```python
from build123d import *

# Parameters (mm, degrees)
SKETCH1_R           = 3.15
BOSS_EXTRUDE1_DEPTH = 12
SKETCH2_R           = 2.1
BOSS_EXTRUDE2_DEPTH = 5


with BuildPart() as part:
    # Sketch1 → Boss-Extrude1 (new body)
    with BuildSketch(Plane(origin=(0, 0, 0), x_dir=(0, 0, -1), z_dir=(1, 0, 0))):
        with BuildLine():
            Line((-15.5, -6), (15.5, -6))
            ThreePointArc((15.5, -6), (16.914213562, -5.414213562), (17.5, -4))
            Line((17.5, -4), (17.5, 4))
            ThreePointArc((17.5, 4), (16.914213562, 5.414213562), (15.5, 6))
            Line((15.5, 6), (-15.5, 6))
            ThreePointArc((-15.5, 6), (-16.914213562, 5.414213562), (-17.5, 4))
            Line((-17.5, 4), (-17.5, -4))
            ThreePointArc((-17.5, -4), (-16.914213562, -5.414213562), (-15.5, -6))
        make_face()
        with Locations((-11.8, 0)):
            Circle(SKETCH1_R, mode=Mode.SUBTRACT)
        with Locations((11.8, 0)):
            Circle(SKETCH1_R, mode=Mode.SUBTRACT)
    extrude(amount=BOSS_EXTRUDE1_DEPTH)

    # Sketch2 → Boss-Extrude2 (add)
    with BuildSketch(Plane.XY):
        with BuildLine():
            Line((30.012822222, 25.164048641), (8.191520443, -6))
            Line((8.191520443, -6), (0, -0.264235636))
            Line((0, -0.264235636), (21.82130178, 30.899813004))
            ThreePointArc((21.82130178, 30.899813004), (23.112309513, 31.722275638), (24.606758741, 31.39096422))
            Line((24.606758741, 31.39096422), (29.521671007, 27.949505602))
            ThreePointArc((29.521671007, 27.949505602), (30.34413364, 26.658497869), (30.012822222, 25.164048641))
        make_face()
        with Locations((24.769909128, 26.393626734)):
            Circle(SKETCH2_R, mode=Mode.SUBTRACT)
        with Locations((20.978568884, 20.979031721)):
            Circle(SKETCH2_R, mode=Mode.SUBTRACT)
        with Locations((17.18722864, 15.564436709)):
            Circle(SKETCH2_R, mode=Mode.SUBTRACT)
        with Locations((13.395888395, 10.149841696)):
            Circle(SKETCH2_R, mode=Mode.SUBTRACT)
    extrude(amount=BOSS_EXTRUDE2_DEPTH)


solid = part.part
```
Here's how the part is built. I have some questions about the finished solid (model axes, mm). Give positions to 0.01 mm unless a question says otherwise; leave off trailing zeros. Order: outer loops, then holes, each group sorted by start corner. A loop starts at its lowest first (then second) coordinate and runs counter-clockwise, first axis right, second up. Notation, with made-up numbers: (41.25, 22.25) - (94.25, 22.25) arc R32 ccw to (94.25, 51.25) - close; hole circle Ø10 at (37.5, 26.25). An arc over 180 degrees is marked (long way). Answer as a JSON object with one key per item and string values. Group by question number.
Item 1: If we section it at A-A on z = 11.8: Please give me the cut outline in (x, y).
Item 2: If we section it at B-B on x = 2: Please give me the cut outline in (y, z).
Item 3: If we mould it in two halves opening along Y, with no side actions, what happens to faces 1 (the cylindrical face through (18.88, 21.07, 2.46)), 2 (the cylindrical face through (23.09, 31.72, 2.46)), 3 (the flat face through (19, 17, 0))? For each: pulls with the +Y half, pulls with the -Y half, needs draft (parallel to the pull), parting line crosses it, or undercut.
Item 4: If we section it at D-D on z = 3.5: Please give me the cut outline in (x, y).
Item 5: Please list where these lines run through material, in increasing order: probe 1 along Y at (x, z) = (4.75, -11.8); probe 2 along Y at (x, z) = (8, -6); probe 3 along Z at (x, y) = (10, 11).
Item 6: If we section it at C-C on y = 17: Please give me the cut outline in (x, z).
Item 7: For P1, Ø6, axis at x = 15.5, y = 22, coming from the +Z side; P2, Ø8, axis at x = 10.5, z = 6, coming from the +Y side; P3, Ø4, axis at x = 13.4, y = 10.15, coming from the -Z side; P4, Ø2, axis at x = 23, y = 23, coming from the -Z side, each with a flat end and sliding along its axis, tell me the tip position at first contact or that it passes through.
Result set:
{
 "1": {"outline": "(0, -6) - (12, -6) - (12, -3.15) - (0, -3.15) - close; (0, 3.15) - (12, 3.15) - (12, 6) - (0, 6) - close"},
 "2": {"outline": "(-6, -15.5) arc R2 ccw to (-4, -17.5) - (4, -17.5) arc R2 ccw to (6, -15.5) - (6, 15.5) arc R2 ccw to (4, 17.5) - (-4, 17.5) arc R2 ccw to (-6, 15.5) - close; hole circle Ø6.3 at (0, -11.8); hole circle Ø6.3 at (0, 11.8)"},
 "3": {"face 1": "undercut", "face 2": "pulls with the +Y half", "face 3": "needs draft"},
 "4": {"outline": "(0, -6) - (12, -6) - (12, -0.56) - (30.01, 25.16) arc R2 ccw to (29.52, 27.95) - (24.61, 31.39) arc R2 ccw to (21.82, 30.9) - (4.39, 6) - (0, 6) - close; hole circle Ø4.2 at (13.4, 10.15); hole circle Ø4.2 at (17.19, 15.56); hole circle Ø4.2 at (20.98, 20.98); hole circle Ø4.2 at (24.77, 26.39)"},
 "5": {"probe 1": "-6 to -3.15, 3.15 to 6", "probe 2": "-6 to 6", "probe 3": "0 to 5"},
 "6": {"outline": "(12.09, 0) - (15.65, 0) - (15.65, 5) - (12.09, 5) - close; (18.72, 0) - (24.3, 0) - (24.3, 5) - (18.72, 5) - close"},
 "7": {"P1": "z = 5", "P2": "y = 20.26", "P3": "through", "P4": "z = 0"}
}
